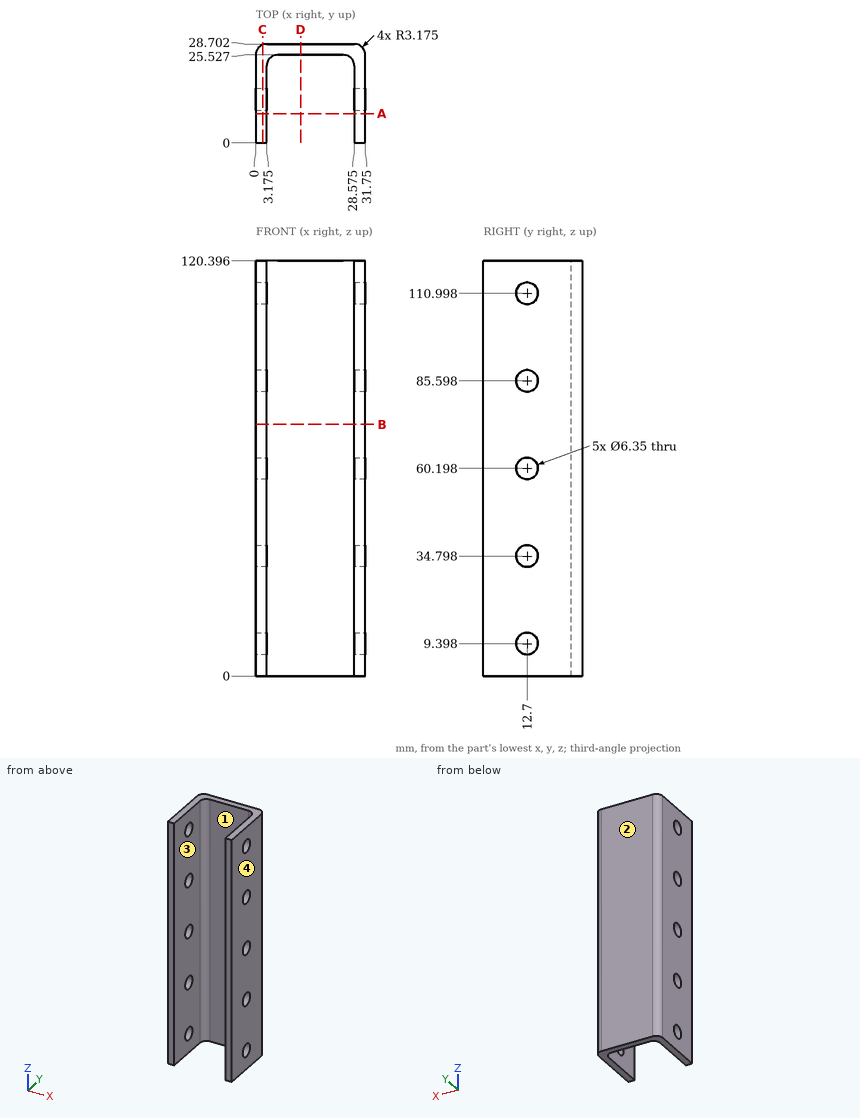
Study the drawing (mm; zero at the part's minimum x, y, z) and answer. Give positions to 0.01 mm unless a question says otherwise; leave off trailing zeros. Write each loop counter-clockwise with the first axis right and the second up, starting at its lowest first coordinate (ties: lowest second). Pieces come first, ordered by that corner, then holes. Notation, with made-up numbers: (53.5, -39) -> (62.5, -39) arc R18 ccw to (62.5, -19) -> close; hole circle Ø8 at (57.5, 45). An arc over 180 degrees is marked (long way). Answer as a JSON object with one key per item and string values. Group by question number.
1) The mould has two halves that part along X. Classify the marked faces 1, 2, 3 and 4: +X half, -X half, draft (parallel to the pull), parting line (faces both ways), or undercut.
2) Find section D-D (x = 13). Write down the section's boundary in (y, z), and give its area (3 significant figures).
3) Find section C-C (x = 2). Write down the section's boundary in (y, z) (3 decimals), and give its area (3 significant figures).
4) Find section B-B (z = 73). Write down the section's boundary in (x, y) (3 decimals), and give its area (3 significant figures).
5) Each of these flat-tipped pins is pushed along its axis until it touches: P1, Ø8.5, axis at y = 12.7, z = 110.998, coming from the -X side; P2, Ø15, axis at x = 12, z = 46.5, coming from the -Y side; P3, Ø3, axis at x = 20, z = 78.5, coming from the -Y side. Where does it stop, or does it pass through?
6) Find section A-A (y = 8.5). Write down the section's boundary in (x, z) (3 decimals), and give its area (3 significant figures).
7) Consider L1, parallel to Z at x = 29.8, y = 12.7; L2, parallel to X at y = 2, z = 105.5 (3 decimals); L3, parallel to Y at x = 17.5, z = 78. Determine where each line is inside the solid, lowest interval first. Write a range as from..to.
Values follow:
{
 "1": {"face 1": "undercut", "face 2": "draft", "face 3": "undercut", "face 4": "+X half"},
 "2": {"outline": "(25.53, 0) -> (28.7, 0) -> (28.7, 120.4) -> (25.53, 120.4) -> close", "area": "382 mm2"},
 "3": {"outline": "(0, 0) -> (28.477, 0) -> (28.477, 120.396) -> (0, 120.396) -> close; hole circle Ø6.35 at (12.7, 9.398); hole circle Ø6.35 at (12.7, 34.798); hole circle Ø6.35 at (12.7, 60.198); hole circle Ø6.35 at (12.7, 85.598); hole circle Ø6.35 at (12.7, 110.998)", "area": "3,270 mm2"},
 "4": {"outline": "(0, 0) -> (3.175, 0) -> (3.175, 22.352) arc R3.175 cw to (6.35, 25.527) -> (25.4, 25.527) arc R3.175 cw to (28.575, 22.352) -> (28.575, 0) -> (31.75, 0) -> (31.75, 25.527) arc R3.175 ccw to (28.575, 28.702) -> (3.175, 28.702) arc R3.175 ccw to (0, 25.527) -> close", "area": "263 mm2"},
 "5": {"P1": "stops at x = 0", "P2": "stops at y = 24.93", "P3": "stops at y = 25.53"},
 "6": {"outline": "(0, 0) -> (3.175, 0) -> (3.175, 120.396) -> (0, 120.396) -> close; (28.575, 0) -> (31.75, 0) -> (31.75, 120.396) -> (28.575, 120.396) -> close", "area": "765 mm2"},
 "7": {"L1": "z = 0..6.22, 12.57..31.62, 37.97..57.02, 63.37..82.42, 88.77..107.82, 114.17..120.4", "L2": "x = 0..3.175, 28.575..31.75", "L3": "y = 25.53..28.7"}
}
